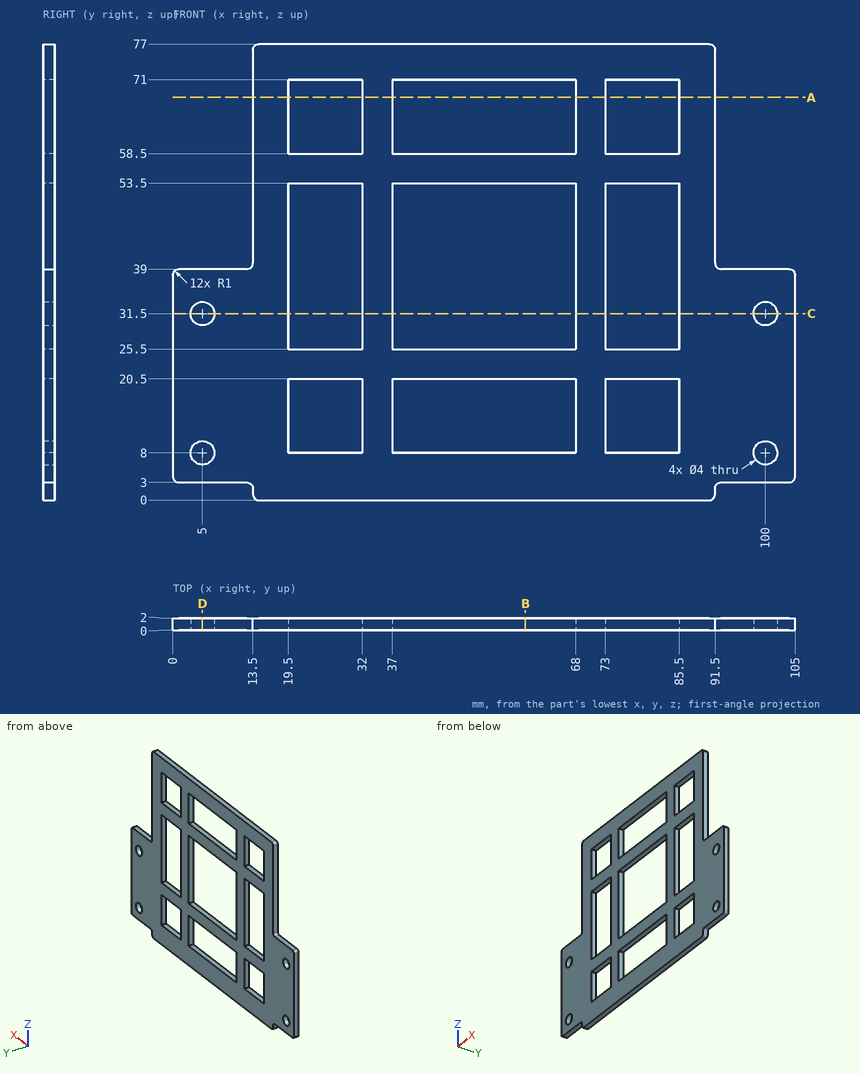
Study the drawing (mm; zero at the part's minimum x, y, z) and answer. Round coordinates to 2 decimals unless told otherwise and drop trailing zeros. Write each loop counter-clockwise with the first axis right and the second up, starting at its lowest first coordinate (ties: lowest second). Pieces come first, ordered by that corner, then holes. Notation, with made-up numbers: (74.25, -15.5) -> (90.25, -15.5) arc R29 ccw to (90.25, 20.5) -> close; hole circle Ø4 at (83, 82). An arc over 180 degrees is marked (long way). Answer as CSV lines item,"result". Start each with the question number.
(1) Find the intervals of material crossed by probe 1 along Z at (x, y) = (100, 1.2); probe 2 along X at (y, z) = (1.35, 31.5); probe 3 along X at (y, z) = (1.3, 47.5), in increasing order.
(2) The part is cut by section D-D, the plane x = 5. Give the vertices of the cut face in (y, z), then the cut area to 3 significant figures.
(3) Each of these flat-tipped pins is pushed along its axis until it touches: pin 1 (8 mm diameter, centred on x = 61.5, z = 40.5, fed in from -Y); pin 2 (0.8 mm diameter, centred on y = 1, z = 1.5, fed in from +X); pin 3 (0.5 mm diameter, centred on y = 0.5, z = 1.5, fed in from -X). Where does it stop, or does it pass through?
(4) The part is cut by section B-B, the plane x = 59.5. Give the vertices of the cut face in (y, z).
(5) The part is cut by section C-C, the plane z = 31.5. Give the vertices of the cut face in (x, y), then the cut area to 3 significant figures.
(6) The part is cut by section A-A, the plane z = 68. Give the vertices of the cut face in (x, y), then the cut area to 3 significant figures.
Output values:
1,probe 1,"z = 3 to 6, 10 to 29.5, 33.5 to 39"
1,probe 2,"x = 0 to 3, 7 to 19.5, 32 to 37, 68 to 73, 85.5 to 98, 102 to 105"
1,probe 3,"x = 13.5 to 19.5, 32 to 37, 68 to 73, 85.5 to 91.5"
2,outline,"(0, 3) -> (2, 3) -> (2, 6) -> (0, 6) -> close; (0, 10) -> (2, 10) -> (2, 29.5) -> (0, 29.5) -> close; (0, 33.5) -> (2, 33.5) -> (2, 39) -> (0, 39) -> close"
2,area,"56.0 mm²"
3,pin 1,"passes through"
3,pin 2,"stops at x = 91.5"
3,pin 3,"stops at x = 13.5"
4,outline,"(0, 0) -> (2, 0) -> (2, 8) -> (0, 8) -> close; (0, 20.5) -> (2, 20.5) -> (2, 25.5) -> (0, 25.5) -> close; (0, 53.5) -> (2, 53.5) -> (2, 58.5) -> (0, 58.5) -> close; (0, 71) -> (2, 71) -> (2, 77) -> (0, 77) -> close"
5,outline,"(0, 0) -> (3, 0) -> (3, 2) -> (0, 2) -> close; (7, 0) -> (19.5, 0) -> (19.5, 2) -> (7, 2) -> close; (32, 0) -> (37, 0) -> (37, 2) -> (32, 2) -> close; (68, 0) -> (73, 0) -> (73, 2) -> (68, 2) -> close; (85.5, 0) -> (98, 0) -> (98, 2) -> (85.5, 2) -> close; (102, 0) -> (105, 0) -> (105, 2) -> (102, 2) -> close"
5,area,"82.0 mm²"
6,outline,"(13.5, 0) -> (19.5, 0) -> (19.5, 2) -> (13.5, 2) -> close; (32, 0) -> (37, 0) -> (37, 2) -> (32, 2) -> close; (68, 0) -> (73, 0) -> (73, 2) -> (68, 2) -> close; (85.5, 0) -> (91.5, 0) -> (91.5, 2) -> (85.5, 2) -> close"
6,area,"44.0 mm²"
